Can you work these out from the drawing? Everything is in mm from the part's minimum corner. A direction names the side the tool comes from. Coordinates: 2 decimals unless noted, no trailing zeros. Write each loop counter-clockwise with the first axis right and the second up, starting at its lowest first coordinate (ties: lowest second). Pieces come first, ordered by that corner, then holes.
(1) Which directions (+Z, -Z, +X, -X, +Y, -Y) give clear straight access to the entire face, cutting with the end or side of a thin tool? Please do the marked faces 1 and 2.
(2) Please list where these lines run through material, in increasing order: probe 1 along Z at (x, y) = (47, 1.55); probe 2 along X at (y, z) = (0.95, 37.3); probe 3 along Y at (x, z) = (39.5, 4.5).
(3) Imagine slicing it at C-C, the plane x = 37.5. List the corners of the cut face in (y, z) for me.
(4) Imagine slicing it at A-A, the plane x = 17.2. List the corners of the cut face in (y, z) for me, plus the area to 3 significant figures.
(5) Imagine slicing it at B-B, the plane z = 2.7. List the corners of the cut face in (x, y) for me, plus the area to 3 significant figures.
(6) Imagine slicing it at D-D, the plane z = 26. List the corners of the cut face in (x, y) for me, plus the area to 3 significant figures.
(7) For pin 1 Ø1.5 at (y, z) = (1, 23.5) entering from -X; pin 2 Ø3.5 at (x, z) = (1.5, 25) entering from -Y; pin 3 Ø2.5 at (y, z) = (1, 25) entering from +X, each with a flat end and sliding along its axis, tell me the tip position at first contact or that it passes through.
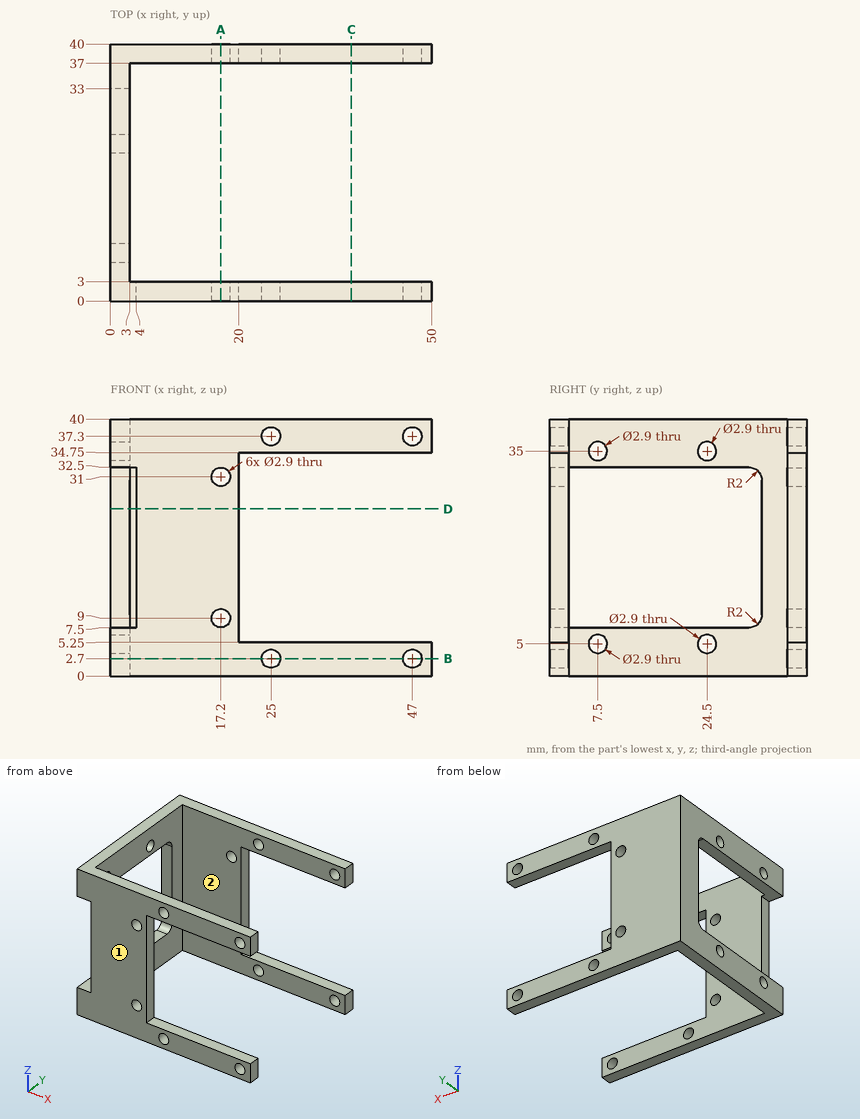
Recorded:
1. face 1: +Z, -Z, +X, -X, -Y
1. face 2: +Z, -Z, +X
2. probe 1: z = 0 to 1.25, 4.15 to 5.25, 34.75 to 35.85, 38.75 to 40
2. probe 2: x = 0 to 23.55, 26.45 to 45.55, 48.45 to 50
2. probe 3: y = 0 to 3, 37 to 40
3. outline: (0, 0) - (3, 0) - (3, 5.25) - (0, 5.25) - close; (0, 34.75) - (3, 34.75) - (3, 40) - (0, 40) - close; (37, 0) - (40, 0) - (40, 5.25) - (37, 5.25) - close; (37, 34.75) - (40, 34.75) - (40, 40) - (37, 40) - close
4. outline: (0, 0) - (3, 0) - (3, 7.55) - (0, 7.55) - close; (0, 10.45) - (3, 10.45) - (3, 29.55) - (0, 29.55) - close; (0, 32.45) - (3, 32.45) - (3, 40) - (0, 40) - close; (37, 0) - (40, 0) - (40, 7.55) - (37, 7.55) - close; (37, 10.45) - (40, 10.45) - (40, 29.55) - (37, 29.55) - close; (37, 32.45) - (40, 32.45) - (40, 40) - (37, 40) - close
4. area: 205 mm2
5. outline: (0, 0) - (23.55, 0) - (23.55, 3) - (3, 3) - (3, 37) - (23.55, 37) - (23.55, 40) - (0, 40) - close; (26.45, 0) - (45.55, 0) - (45.55, 3) - (26.45, 3) - close; (26.45, 37) - (45.55, 37) - (45.55, 40) - (26.45, 40) - close; (48.45, 0) - (50, 0) - (50, 3) - (48.45, 3) - close; (48.45, 37) - (50, 37) - (50, 40) - (48.45, 40) - close
5. area: 367 mm2
6. outline: (0, 33) - (3, 33) - (3, 37) - (20, 37) - (20, 40) - (0, 40) - close; (4, 0) - (20, 0) - (20, 3) - (4, 3) - close
6. area: 120 mm2
7. pin 1: stops at x = 4
7. pin 2: stops at y = 33
7. pin 3: stops at x = 20
